Model file for the job. Use its own axes, mm. Face numbers are marked on the shaded views. Round coordinates to 2 decimals unless told otherwise and drop trailing zeros. Loops run counter-clockwise (first coordinate to the right, second up) from the corner with the lowest first, then second, coordinate; pieces in that order, holes last. Notation, with made-up numbers: (5.25, 12.5) -> (61.25, 12.5) arc R32 cw to (61.25, 38.5) -> close; hole circle Ø4 at (-36.5, 80). An arc over 180 degrees is marked (long way). Use a Markdown table: item, result. Add a question column.
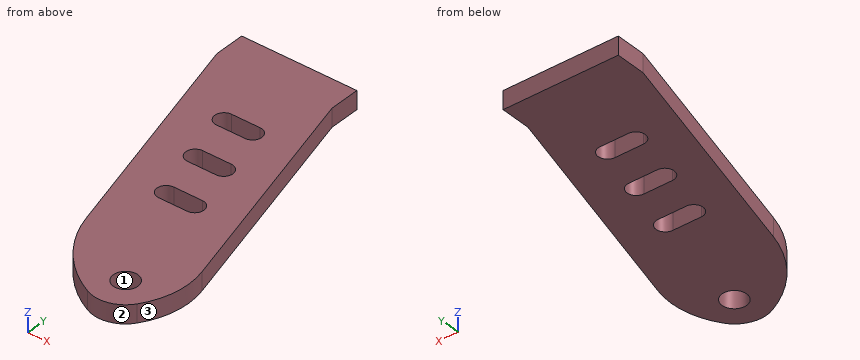
```python
from build123d import *

# Parameters (mm, degrees)
SKETCH1_R           = 4.05
BOSS_EXTRUDE1_DEPTH = 6


with BuildPart() as part:
    # Sketch1 → Boss-Extrude1 (new body)
    with BuildSketch(Plane.XY):
        with BuildLine():
            Line((0, 0), (38, 0))
            Line((38, 0), (38, -10))
            Line((38, -10), (57.980052552, -87))
            ThreePointArc((57.980052552, -87), (58.395271252, -98.14362649), (54.093497988, -108.431851056))
            ThreePointArc((54.093497988, -108.431851056), (48.062167082, -112.638750827), (40.737765228, -111.984460623))
            ThreePointArc((40.737765228, -111.984460623), (27.569508693, -101.809733527), (19.980052552, -87))
            Line((19.980052552, -87), (0, -10))
            Line((0, -10), (0, 0))
        make_face()
        with Locations((45.2987713, -102.25)):
            Circle(SKETCH1_R, mode=Mode.SUBTRACT)
        with BuildLine():
            Line((24.290026276, -45.45), (33.690026276, -45.45))
            ThreePointArc((33.690026276, -45.45), (36.740026276, -48.5), (33.690026276, -51.55))
            Line((33.690026276, -51.55), (24.290026276, -51.55))
            ThreePointArc((24.290026276, -51.55), (21.240026276, -48.5), (24.290026276, -45.45))
        make_face(mode=Mode.SUBTRACT)
        with BuildLine():
            Line((28.72715483, -62.55), (38.12715483, -62.55))
            ThreePointArc((38.12715483, -62.55), (41.17715483, -65.6), (38.12715483, -68.65))
            Line((38.12715483, -68.65), (28.72715483, -68.65))
            ThreePointArc((28.72715483, -68.65), (25.67715483, -65.6), (28.72715483, -62.55))
        make_face(mode=Mode.SUBTRACT)
        with BuildLine():
            Line((19.852897722, -28.35), (29.252897722, -28.35))
            ThreePointArc((29.252897722, -28.35), (32.302897722, -31.4), (29.252897722, -34.45))
            Line((29.252897722, -34.45), (19.852897722, -34.45))
            ThreePointArc((19.852897722, -34.45), (16.802897722, -31.4), (19.852897722, -28.35))
        make_face(mode=Mode.SUBTRACT)
    extrude(amount=BOSS_EXTRUDE1_DEPTH)


solid = part.part
```
1) Cut at C-C on y = -102.25. Write the cut outline in (x, z), and give its area (3 significant figures).
2) Pull direction Y, two halves, no side cores. Call the marked faces 1, 2 and 3: +Y half, -Y half, draft (parallel to the pull), parting line (faces both ways), or undercut.
3) Cut at B-B on y = -48.5. Write the cut outline in (x, z).
4) Cut at A-A on z = 2.4. Write the cut outline in (x, y).
5) Wall check: probe 1 along Y at (x, z) = (30.5, 4.3); probe 2 along Y at (x, z) = (30, 3.3); probe 3 along Y at (x, z) = (37, 0.6). Give the ranges that are in metal, low to high. Write a range as from..to.
6) Pin check, flat tips, straight feed: pin 1 Ø5 at (x, y) = (51.5, -47.5) entering from -Z; pin 2 Ø3 at (x, z) = (28, 3) entering from +Y; pin 3 Ø3 at (x, z) = (34, 2.5) entering from -Y; pin 4 Ø1 at (y, z) = (-88, 4.5) entering from +X. Stop position of each tip, or through.
7) Cut at D-D on x = 10. Write the cut outline in (y, z).
Established:
| question | item | result |
|---|---|---|
| 1 | outline | (27.94, 0) -> (41.25, 0) -> (41.25, 6) -> (27.94, 6) -> close; (49.35, 0) -> (57.3, 0) -> (57.3, 6) -> (49.35, 6) -> close |
| 1 | area | 128 mm^2 |
| 2 | face 1 | undercut |
| 2 | face 2 | -Y half |
| 2 | face 3 | parting line |
| 3 | outline | (9.99, 0) -> (21.24, 0) -> (21.24, 6) -> (9.99, 6) -> close; (36.74, 0) -> (47.99, 0) -> (47.99, 6) -> (36.74, 6) -> close |
| 4 | outline | (0, -10) -> (19.98, -87) arc R38.18 ccw to (40.74, -111.98) arc R10.75 ccw to (54.09, -108.43) arc R25.94 ccw to (57.98, -87) -> (38, -10) -> (38, 0) -> (0, 0) -> close; hole (19.85, -34.45) -> (29.25, -34.45) arc R3.05 ccw to (29.25, -28.35) -> (19.85, -28.35) arc R3.05 ccw to start; hole (24.29, -51.55) -> (33.69, -51.55) arc R3.05 ccw to (33.69, -45.45) -> (24.29, -45.45) arc R3.05 ccw to start; hole (28.73, -68.65) -> (38.13, -68.65) arc R3.05 ccw to (38.13, -62.55) -> (28.73, -62.55) arc R3.05 ccw to start; hole circle Ø8.1 at (45.3, -102.25) |
| 5 | probe 1 | y = -104.96..-68.65, -62.55..-51.55, -45.45..-34.18, -28.62..0 |
| 5 | probe 2 | y = -104.47..-68.65, -62.55..-51.55, -45.45..-34.36, -28.44..0 |
| 5 | probe 3 | y = -109.97..-68.65, -62.55..0 |
| 6 | pin 1 | passes through |
| 6 | pin 2 | stops at y = 0 |
| 6 | pin 3 | stops at y = -109.01 |
| 6 | pin 4 | stops at x = 58.32 |
| 7 | outline | (-48.54, 0) -> (0, 0) -> (0, 6) -> (-48.54, 6) -> close |
